Read the model definition and answer for the solid it produces. Units are mm, in the model's axes. A direction names the side the tool comes from. Round coordinates to 2 decimals unless told otherwise and drop trailing zeros. Write each loop counter-clockwise with the first axis right and the second up, starting at its lowest first coordinate (ties: lowest second). Pieces come first, ordered by that corner, then holes. Notation, with made-up numbers: (1.5, 5) - (53.5, 5) arc R19 cw to (53.5, 30) - close; hole circle Ø8 at (33.25, 83). An arc over 180 degrees is marked (long way). Use one line per item in the form item = value. Start each with the question number.
1) The part is cut by section D-D, the plane y = -38.1. Give the vertices of the cut face in (x, z), plus the area to 3 significant figures.
2) Each of these flat-tipped pins is pushed along its axis until it touches: pin 1 (4 mm diameter, centred on x = -10.5, y = -27, fed in from +Z); pin 2 (6 mm diameter, centred on x = -16, y = -53.5, fed in from -Z); pin 3 (12 mm diameter, centred on x = -8.5, y = -97, fed in from +Z). Where does it stop, or does it pass through?
3) For a pull along Y with two mould halves and no side action, classify faces 3 (the face through (0, 0, 0)), 4 (the face through (5.866, -15.132, -0.178)), 5 (the face through (-15.12, -81.42, -11.59)) as released by +Y, released by -Y, zero draft, split by the parting line, or undercut.
4) Consider line 1 along Y through (x, z) = (0, 0.25); line 2 along Y through (x, z) = (-2.5, 3); line 3 along X through (y, z) = (-12.7, 7.25). Determine where each line is inside the solid, lowest interval first. Write a range as from..to.
5) The part is cut by section C-C, the plane y = -65. Give the vertices of the cut face in (x, z), plus the area to 3 significant figures.
6) The part is cut by section A-A, the plane z = 0. Count the separate pieces of the cut face and the enclosed holes in it, plus the area to 3 significant figures.
7) For faces 1 (the face through (6.827, -25.044, 10.709)), 2 (the face through (5.866, -40.532, -0.178)), determine the directions among +Z, -Z, +X, -X, +Y, -Y from which every point of the face is accessible in a straight line to the end or side of a thin tool.
from build123d import *

# Parameters (mm, degrees)
F0_R          = 12.7
F1_DEPTH      = 50.8
F2_R          = 19.05
F3_DEPTH      = 50.8
F4_R          = 31.75
F5_DEPTH      = 25.4
F6_R          = 6.35
F7_DEPTH      = 12.7
F7_DEPTH_BACK = 12.7
F8_R          = 6.35
F9_DEPTH      = 12.7
F9_DEPTH_BACK = 12.7
F13_R         = 6.35
F15_S5_R      = 19.05
F15_T6_DEPTH  = 47


# Not quite as in the source:
# - a fillet or chamfer that OpenCascade refuses, or shapes differently, is made with other operations: its cross-section is extruded or revolved along the edge and cut away or added


with BuildPart() as f1:
    # F0 (on Front) → F1 (new body)
    with BuildSketch(Plane.XZ):
        Circle(F0_R)
    extrude(amount=F1_DEPTH)

    # F2 (on face) → F3 (join)
    with BuildSketch(Plane.XZ.offset(50.8)):
        Circle(F2_R)
    extrude(amount=F3_DEPTH)

    # F4 (on face) → F5 (join)
    with BuildSketch(Plane.XZ.offset(101.6)):
        Circle(F4_R)
    extrude(amount=F5_DEPTH)

    # F6 (on Top) → F7 (cut, two sides)
    with BuildSketch(Plane.XY) as f7_sk:
        with Locations((0, -38.1)):
            Circle(F6_R)
    extrude(amount=-F7_DEPTH, mode=Mode.SUBTRACT)
    extrude(f7_sk.sketch, amount=F7_DEPTH_BACK, mode=Mode.SUBTRACT)

    # F8 (on Top) → F9 (cut, two sides)
    with BuildSketch(Plane.XY) as f9_sk:
        with Locations((0, -12.7)):
            Circle(F8_R)
    extrude(amount=-F9_DEPTH, mode=Mode.SUBTRACT)
    extrude(f9_sk.sketch, amount=F9_DEPTH_BACK, mode=Mode.SUBTRACT)

    # F10: fillet of radius 12.7 on 1 edges, made by hand

    # F10_s1 → F10_t2 (revolve, cut)
    with BuildSketch(Plane.XY):
        with BuildLine():
            ThreePointArc((19.05, -61.7985226281), (17.3485226281, -55.4485226281), (12.7, -50.8))
            Line((12.7, -50.8), (19.05, -50.8))
            Line((19.05, -50.8), (19.05, -61.7985226281))
        make_face()
    revolve(axis=Axis((0, -50.8, 0), (0, -1, 0)), mode=Mode.SUBTRACT)

    # F14: sweep along a path in F12
    with BuildLine(Plane.XZ.offset(114.3)) as f14_path:
        CenterArc((0, 0), 31.75, 0, 360)
    # F13 (on Right) → F14 (sweep, cut)
    with BuildSketch(Plane.YZ):
        with Locations((-114.3, 31.75)):
            Circle(F13_R)
    sweep(path=f14_path.line, mode=Mode.SUBTRACT)

    # F15: chamfer of 12.7 on 1 edges, made by hand


with BuildPart() as f15_tool2:
    # F15_s3 → F15_t4 (revolve)
    with BuildSketch(Plane.XY):
        Polygon((31.75, -114.3), (19.05, -101.6), (31.75, -101.6), align=None)
    revolve(axis=Axis((0, -101.6, 0), (0, -1, 0)))

    # F15_s5 → F15_t6 (cut, symmetric)
    with BuildSketch(Plane.XZ.offset(108)):
        Circle(F15_S5_R)
    extrude(amount=F15_T6_DEPTH, both=True, mode=Mode.SUBTRACT)


with BuildPart() as f1_1:
    add(f1.part)

    # F15_t1: cut F15_tool2
    add(f15_tool2.part, mode=Mode.SUBTRACT)


solid = f1_1.part
Geometry results:
q1.outline = (-6.35, -11) - (-6.35, 11) arc R12.7 ccw to start; (6.35, -11) arc R12.7 ccw to (6.35, 11) - close
q1.area = 198 mm2
q2.pin_1 = 9.44
q2.pin_2 = -10.63
q2.pin_3 = 19.03
q3.face_3 = released by +Y
q3.face_4 = undercut
q3.face_5 = zero draft
q4.line_1 = -127..-44.45, -31.75..-19.05, -6.35..0
q4.line_2 = -127..-43.94, -32.26..-18.54, -6.86..0
q4.line_3 = -10.43..-6.35, 6.35..10.43
q5.outline = circle Ø38.1 at (0, 0)
q5.area = 1,140 mm2
q6.separate_pieces = 1
q6.enclosed_holes = 2
q6.area = 4,290 mm2
q7.face_1 = +Y
q7.face_2 = +Z, -Z
